Part model, mm, in its own coordinate system. Face numbers are marked on the shaded views. Coordinates: 2 decimals unless noted, no trailing zeros. Order: outer loops, then holes, each group sorted by start corner. A loop starts at its lowest first (then second) coordinate and runs counter-clockwise, first axis right, second up. Notation, with made-up numbers: (-4.75, 71.5) - (15.25, 71.5) arc R12 cw to (15.25, 90.5) - close; hole circle Ø1 at (-31.75, 13.5). An arc over 180 degrees is marked (long way). Use a Markdown table: item, result. Add a question column.
1) Wall check: L1, parallel to Y at x = 0, z = 1.2; L2, parallel to X at y = -1, z = 3.5; L3, parallel to X at y = -13.5, z = 2.75. Give the ranges that are in metal, low to high. Write a range as [from, to].
2) Two-plate mould, pull along Y, no slides. Class the marked faces 1, 2 and 3: +Y half, -Y half, draft (parallel to the pull), parting line (faces both ways), or undercut.
3) Saw through at A-A on y = 5.5. List the corners of the cut face in (x, z).
4) Drop flat-ended pins along their axis: P1, Ø2, axis at x = -27, y = -24.5, coming from the +Z side; P2, Ø3, axis at x = 26, y = 24, coming from the +Z side; P3, Ø4, axis at x = -28.5, y = 6.5, coming from the +Z side. Give the stop position or say it passes through.
5) Saw through at C-C on x = 22. List the corners of the cut face in (y, z), then the cut area to 3 significant figures.
6) Saw through at B-B on x = -15. List the corners of the cut face in (y, z), then the cut area to 3 significant figures.
7) Saw through at D-D on y = -20. List the corners of the cut face in (x, z).
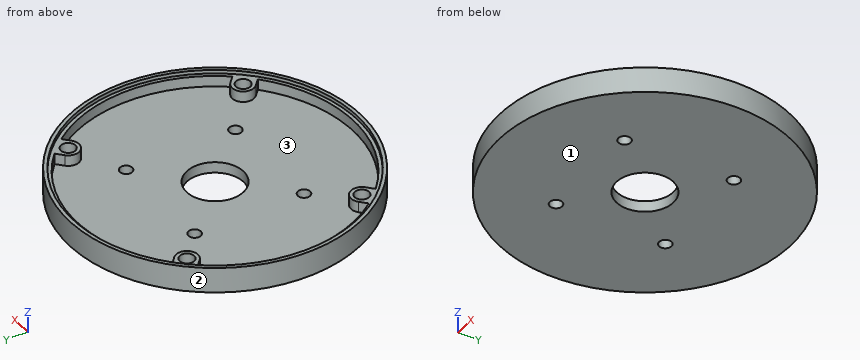
```python
from build123d import *

# Parameters (mm, degrees)
SKETCH_R           = 40
SKETCH_R_2         = 7.8
PAD_DEPTH          = 3
SKETCH001_R        = 1.7
POCKET_DEPTH       = 229.354706
POLARPATTERN_COUNT = 4
SKETCH002_R        = 40
SKETCH002_R_2      = 38
PAD001_DEPTH       = 3
SKETCH003_R        = 40
SKETCH003_R_2      = 39
PAD002_DEPTH       = 1
PAD003_DEPTH       = 3
SKETCH005_R        = 2
POCKET001_DEPTH    = 5


with BuildPart() as part:
    # Sketch → Pad (new body)
    with BuildSketch(Plane.XY):
        Circle(SKETCH_R)
        Circle(SKETCH_R_2, mode=Mode.SUBTRACT)
    extrude(amount=PAD_DEPTH)

    # Sketch001 → Pocket (cut, through all)
    with BuildSketch(Plane.XY.offset(3)):
        with Locations((15, 15)):
            Circle(SKETCH001_R)
    pocket = extrude(amount=-POCKET_DEPTH, mode=Mode.SUBTRACT)

    # PolarPattern: Pocket ×4 about axis
    polarpattern_axis = Axis((0, 0, 3), (0, 0, 1))
    for i in range(1, POLARPATTERN_COUNT):
        add(pocket.rotate(polarpattern_axis, i * 360 / POLARPATTERN_COUNT), mode=Mode.SUBTRACT)

    # Sketch002 → Pad001 (new body)
    with BuildSketch(Plane.XY.offset(3)):
        Circle(SKETCH002_R)
        Circle(SKETCH002_R_2, mode=Mode.SUBTRACT)
    extrude(amount=PAD001_DEPTH)

    # Sketch003 → Pad002 (new body)
    with BuildSketch(Plane.XY.offset(6)):
        Circle(SKETCH003_R)
        Circle(SKETCH003_R_2, mode=Mode.SUBTRACT)
    extrude(amount=PAD002_DEPTH)

    # Sketch004 → Pad003 (new body)
    with BuildSketch(Plane.XY.offset(3)):
        with BuildLine():
            ThreePointArc((23.96516, 26.20441), (23.79559, 21.96516), (28.03484, 21.79559))
            Line((29.957371, 23.570234), (28.03484, 21.79559))
            Line((25.887691, 27.979054), (29.957371, 23.570234))
            Line((23.96516, 26.20441), (25.887691, 27.979054))
        make_face()
        with BuildLine():
            ThreePointArc((28.03484, -21.79559), (23.79559, -21.96516), (23.96516, -26.20441))
            Line((23.96516, -26.20441), (25.887691, -27.979054))
            Line((25.887691, -27.979054), (29.957371, -23.570234))
            Line((29.957371, -23.570234), (28.03484, -21.79559))
        make_face()
    pad003 = extrude(amount=PAD003_DEPTH)

    # Mirrored: Pad003 across Sketch004 V_Axis
    add(pad003.mirror(Plane(origin=(0, 0, 3), x_dir=(0, 0, 1), z_dir=(1, 0, 0))))

    # Sketch005 → Pocket001 (cut)
    with BuildSketch(Plane.XY.offset(6)):
        with Locations((-26, 24)):
            Circle(SKETCH005_R)
        with Locations((-26, -24)):
            Circle(SKETCH005_R)
        with Locations((26, -24)):
            Circle(SKETCH005_R)
        with Locations((26, 24)):
            Circle(SKETCH005_R)
    extrude(amount=-POCKET001_DEPTH, mode=Mode.SUBTRACT)


solid = part.part
```
Results are:
| question | item | result |
|---|---|---|
| 1 | L1 | [-40, -7.8], [7.8, 40] |
| 1 | L2 | [-39.99, -37.99], [37.99, 39.99] |
| 1 | L3 | [-37.65, -15.8], [-14.2, 14.2], [15.8, 37.65] |
| 2 | face 1 | draft |
| 2 | face 2 | parting line |
| 2 | face 3 | undercut |
| 3 | outline | (-39.62, 0) - (-5.53, 0) - (-5.53, 3) - (-37.6, 3) - (-37.6, 6) - (-38.61, 6) - (-38.61, 7) - (-39.62, 7) - close; (5.53, 0) - (39.62, 0) - (39.62, 7) - (38.61, 7) - (38.61, 6) - (37.6, 6) - (37.6, 3) - (5.53, 3) - close |
| 4 | P1 | z = 6 |
| 4 | P2 | z = 1 |
| 4 | P3 | z = 3 |
| 5 | outline | (-33.41, 0) - (33.41, 0) - (33.41, 7) - (32.2, 7) - (32.2, 6) - (30.98, 6) - (30.98, 3) - (-30.98, 3) - (-30.98, 6) - (-32.2, 6) - (-32.2, 7) - (-33.41, 7) - close |
| 5 | area | 217 mm2 |
| 6 | outline | (-37.08, 0) - (-16.7, 0) - (-16.7, 3) - (-34.91, 3) - (-34.91, 6) - (-36, 6) - (-36, 7) - (-37.08, 7) - close; (-13.3, 0) - (13.3, 0) - (13.3, 3) - (-13.3, 3) - close; (16.7, 0) - (37.08, 0) - (37.08, 7) - (36, 7) - (36, 6) - (34.91, 6) - (34.91, 3) - (16.7, 3) - close |
| 6 | area | 217 mm2 |
| 7 | outline | (-34.64, 0) - (34.64, 0) - (34.64, 7) - (33.48, 7) - (33.48, 6) - (32.31, 6) - (32.31, 3) - (-32.31, 3) - (-32.31, 6) - (-33.48, 6) - (-33.48, 7) - (-34.64, 7) - close |
